Design review of the part built by this model. Coordinates are the model's own, in mm. A direction names the side the tool comes from. Coordinates: 2 decimals unless noted, no trailing zeros. Loops run counter-clockwise (first coordinate to the right, second up) from the corner with the lowest first, then second, coordinate; pieces in that order, holes last. Notation, with made-up numbers: (74, 26.5) -> (100, 26.5) arc R31 cw to (100, 58.5) -> close; hole circle Ø5 at (-14.75, 54). An arc over 180 degrees is marked (long way). One line per item, written item: value. Start each with the question number.
1. Add section A-A on x = -9. Write out the cut boundary in (y, z) (3 decimals), plus the area to 3 significant figures.
2. Add section B-B on y = 2. Write out the cut boundary in (x, z) (3 decimals).
3. For probe 1 along Z at (x, y) = (2, 2.25) (3 decimals), list the stretches that pass through material, from the lowest coordinate up.
4. Machinability: for faces 4 (the flat face through (-15.875, 1, 68)), 5 (the flat face through (-1, 0, -1)), which of the approach directions +Z, -Z, +X, -X, +Y, -Y give a long, thin tool a straight path to every point of the face, cutting with its end or side? Answer none if there is none.
5. Draft analysis for pull direction Z (two halves, no side actions). For faces 1 (the flat face through (15.875, 1, 68)), 2 (the flat face through (40.647, 1, 1)), 3 (the flat face through (-1, 1, 73.025)), state which applies: pulls with the +Z half, pulls with the -Z half, needs draft (parallel to the pull), parting line crosses it, or undercut.
```python
from build123d import *

# Parameters (mm, degrees)
SKETCH1_W           = 81.2942748
SKETCH1_H           = 146.05
SKETCH1_W_2         = 31.75
SKETCH1_H_2         = 3.429
SKETCH1_W_3         = 0.79375
SKETCH1_H_3         = 3.556
BOSS_EXTRUDE1_DEPTH = 2.9972


with BuildPart() as part:
    # Sketch1 → Boss-Extrude1 (new body)
    with BuildSketch(Plane(origin=(0, 0, 0), x_dir=(1, 0, 0), z_dir=(0, 1, 0))):
        Rectangle(SKETCH1_W, SKETCH1_H)
        with Locations((0, 68.3387)):
            Rectangle(SKETCH1_W_2, SKETCH1_H_2, mode=Mode.SUBTRACT)
        with Locations((0, -68.3387)):
            Rectangle(SKETCH1_W_2, SKETCH1_H_2, mode=Mode.SUBTRACT)
        with Locations((-36.61676177, -68.2752)):
            Rectangle(SKETCH1_W_3, SKETCH1_H_3, mode=Mode.SUBTRACT)
        with Locations((-35.02926177, -68.2752)):
            Rectangle(SKETCH1_W_3, SKETCH1_H_3, mode=Mode.SUBTRACT)
        with Locations((-33.44176177, -68.2752)):
            Rectangle(SKETCH1_W_3, SKETCH1_H_3, mode=Mode.SUBTRACT)
    extrude(amount=BOSS_EXTRUDE1_DEPTH)


solid = part.part
```
Worked answers:
1. outline: (0, -73.025) -> (2.997, -73.025) -> (2.997, -70.053) -> (0, -70.053) -> close; (0, -66.624) -> (2.997, -66.624) -> (2.997, 66.624) -> (0, 66.624) -> close; (0, 70.053) -> (2.997, 70.053) -> (2.997, 73.025) -> (0, 73.025) -> close
1. area: 417 mm²
2. outline: (-40.647, -73.025) -> (40.647, -73.025) -> (40.647, 73.025) -> (-40.647, 73.025) -> close; hole (-37.014, 66.497) -> (-36.22, 66.497) -> (-36.22, 70.053) -> (-37.014, 70.053) -> close; hole (-35.426, 66.497) -> (-34.632, 66.497) -> (-34.632, 70.053) -> (-35.426, 70.053) -> close; hole (-33.839, 66.497) -> (-33.045, 66.497) -> (-33.045, 70.053) -> (-33.839, 70.053) -> close; hole (-15.875, -70.053) -> (15.875, -70.053) -> (15.875, -66.624) -> (-15.875, -66.624) -> close; hole (-15.875, 66.624) -> (15.875, 66.624) -> (15.875, 70.053) -> (-15.875, 70.053) -> close
3. probe 1: z = -73.025 to -70.053, -66.624 to 66.624, 70.053 to 73.025
4. face 4: +Y, -Y
4. face 5: +Z, -Z, +X, -X, -Y
5. face 1: undercut
5. face 2: needs draft
5. face 3: pulls with the +Z half
